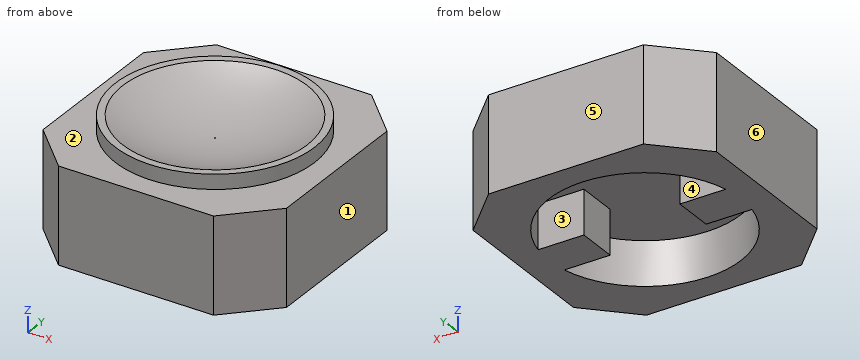
from build123d import *

# Parameters (mm, degrees)
BOSS_EXTRUDE2_DEPTH = 6.5
SKETCH2_R           = 6.25
CUT_EXTRUDE1_DEPTH  = 0.5
BOSS_EXTRUDE6_START = 1
SKETCH8_R           = 6.75
SKETCH8_R_2         = 6.25
BOSS_EXTRUDE6_DEPTH = 1
FILLET5_R           = 13.6
SKETCH3_R           = 6.5
CUT_EXTRUDE2_DEPTH  = 3
SKETCH9_W           = 3.957503607
SKETCH9_H           = 2.75
BOSS_EXTRUDE7_DEPTH = 3


with BuildPart() as part:
    # Sketch1 → Boss-Extrude2 (new body)
    with BuildSketch(Plane.XY):
        Polygon((-8.25, -5.25), (-5.25, -8.25), (5.25, -8.25), (8.25, -5.25), (8.25, 5.25), (5.25, 8.25), (-5.25, 8.25), (-8.25, 5.25), align=None)
    extrude(amount=BOSS_EXTRUDE2_DEPTH)

    # Sketch2 → Cut-Extrude1 (cut)
    with BuildSketch(Plane.XY.offset(6.5)):
        Circle(SKETCH2_R)
    extrude(amount=-CUT_EXTRUDE1_DEPTH, mode=Mode.SUBTRACT)

    # Sketch8 → Boss-Extrude6 (add)
    with BuildSketch(Plane.XY.offset(6.5).offset(BOSS_EXTRUDE6_START)):
        Circle(SKETCH8_R)
        Circle(SKETCH8_R_2, mode=Mode.SUBTRACT)
    extrude(amount=-BOSS_EXTRUDE6_DEPTH)

    # Fillet5
    # the kernel refuses this fillet: 13.6 mm, written as the material it adds along each edge
    with BuildSketch(Plane(origin=(0, 0, 6), x_dir=(1, 0, 0), z_dir=(0, -1, 0))) as fillet5_piece_1:
        with BuildLine():
            CenterArc((0.041135369, 13.6), FILLET5_R, 270, 27.163688564)
            Line((0.041135369, 0), (0.041135369, -0.272))
            Line((0.041135369, -0.272), (6.25, -0.272))
            Line((6.25, -0.272), (6.522, 0))
            ThreePointArc((6.522, 0), (6.522, 0.75), (6.374177293, 1.258))
            Line((6.374177293, 1.258), (6.25, 1.5))
        make_face()
    revolve(axis=Axis((0, 0, 6), (0, 0, 1)))

    # Sketch3 → Cut-Extrude2 (cut)
    with BuildSketch(Plane(origin=(0, 0, 0), x_dir=(-1, 0, 0), z_dir=(0, 0, -1))):
        Circle(SKETCH3_R)
    extrude(amount=-CUT_EXTRUDE2_DEPTH, mode=Mode.SUBTRACT)

    # Sketch9 → Boss-Extrude7 (add)
    with BuildSketch(Plane(origin=(0, 0, 3), x_dir=(-1, 0, 0), z_dir=(0, 0, -1))):
        with Locations((-5.228751803, 0)):
            Rectangle(SKETCH9_W, SKETCH9_H)
        with Locations((5.228751803, 0)):
            Rectangle(SKETCH9_W, SKETCH9_H)
    extrude(amount=BOSS_EXTRUDE7_DEPTH)


solid = part.part
Source: CAD feature listing. Evaluate the final solid. Frame: model axes, mm. Face numbers are marked on the shaded views. A direction names the side the tool comes from. Give positions to 0.01 mm unless a question says otherwise; leave off trailing zeros. Write each loop counter-clockwise with the first axis right and the second up, starting at its lowest first coordinate (ties: lowest second). Pieces come first, ordered by that corner, then holes. Notation, with made-up numbers: M 59,23.5 L 95,23.5 A21 cw 95,31.5 Z; hole C -25.5,64 d5. An arc over 180 degrees is marked long. Return JSON: item names as keys, results as strings. Group by question number.
1) Set-up query: the marked faces 1, 2 and 3. Return all of +Z, -Z, +X, -X, +Y, -Y with unobstructed straight access to the full face (end or side cutting, diameter ignored); none if empty.
2) Cut plane B-B, the plane z = 5.5. Output: boundary loops of the cut face in (x, y).
3) Draft query along X for the marked faces 4, 5 and 6. Return one class per face: released by +X, released by -X, zero draft, split by the parting line, or undercut.
4) Ray query, L1, parallel to Z at x = -1.5, y = -2.75; L2, parallel to Z at x = -6.5, y = -5; L3, parallel to Y at x = -7, z = 3.5. Return the intervals inside material, ascending.
5) Cut plane A-A, the plane z = 2.5. Output: boundary loops of the cut face in (x, y) (3 decimals), then the cut area to 3 significant figures.
Data:
{
 "1": {"face 1": "+Z, -Z, +X, +Y, -Y", "face 2": "+Z", "face 3": "-Z"},
 "2": {"outline": "M -8.25,-5.25 L -5.25,-8.25 L 5.25,-8.25 L 8.25,-5.25 L 8.25,5.25 L 5.25,8.25 L -5.25,8.25 L -8.25,5.25 Z"},
 "3": {"face 4": "undercut", "face 5": "zero draft", "face 6": "released by -X"},
 "4": {"L1": "z = 3 to 6.36", "L2": "z = 0 to 6.5", "L3": "y = -6.5 to 6.5"},
 "5": {"outline": "M -8.25,-5.25 L -5.25,-8.25 L 5.25,-8.25 L 8.25,-5.25 L 8.25,5.25 L 5.25,8.25 L -5.25,8.25 L -8.25,5.25 Z; hole M -6.353,-1.375 A6.5 ccw 6.353,-1.375 L 3.25,-1.375 L 3.25,1.375 L 6.353,1.375 A6.5 ccw -6.353,1.375 L -3.25,1.375 L -3.25,-1.375 Z", "area": "139 mm²"}
}
